Here's how the part is built. I have some questions about the finished solid (model axes, mm). Coordinates: 2 decimals unless noted, no trailing zeros. Write each loop counter-clockwise with the first axis right and the second up, starting at its lowest first coordinate (ties: lowest second). Pieces come first, ordered by that corner, then holes. Notation, with made-up numbers: M -17.75,-4.75 L -1.75,-4.75 A33 ccw -1.75,28.25 Z; hole C 63,69.5 d7. An arc over 180 degrees is marked long. Use a Markdown table: item, result.
```python
from build123d import *

# Parameters (mm, degrees)
F0_R     = 30
F0_R_2   = 2.5
F1_DEPTH = 6


with BuildPart() as f1:
    # F0 (on Top) → F1 (new body)
    with BuildSketch(Plane.XY):
        Circle(F0_R)
        with Locations((-11.5, -8.75)):
            Circle(F0_R_2, mode=Mode.SUBTRACT)
        with Locations((0, -8.75)):
            Circle(F0_R_2, mode=Mode.SUBTRACT)
        with Locations((11.5, -8.75)):
            Circle(F0_R_2, mode=Mode.SUBTRACT)
        with Locations((-11.5, 8.75)):
            Circle(F0_R_2, mode=Mode.SUBTRACT)
        with Locations((0, 8.75)):
            Circle(F0_R_2, mode=Mode.SUBTRACT)
        with Locations((11.5, 8.75)):
            Circle(F0_R_2, mode=Mode.SUBTRACT)
    extrude(amount=F1_DEPTH)


solid = f1.part
```
1. Suppose I cut it at D-D on x = 13. Write out the boundary of the cut face in (y, z), and give its area (3 significant figures).
Answers follow:
| item | result |
|---|---|
| outline | M -27.04,0 L -10.75,0 L -10.75,6 L -27.04,6 Z; M -6.75,0 L 6.75,0 L 6.75,6 L -6.75,6 Z; M 10.75,0 L 27.04,0 L 27.04,6 L 10.75,6 Z |
| area | 276 mm2 |
2. I need wall thicknesses on probe 1 along Y at (x, z) = (0, 3.6); probe 2 along X at (y, z) = (8, 0.8); probe 3 along Y at (x, z) = (-9.5, 3.6). Which ranges of each line are inside material? Lowest first, please.
Answers follow:
| item | result |
|---|---|
| probe 1 | y = -30 to -11.25, -6.25 to 6.25, 11.25 to 30 |
| probe 2 | x = -28.91 to -13.88, -9.12 to -2.38, 2.38 to 9.12, 13.88 to 28.91 |
| probe 3 | y = -28.46 to -10.25, -7.25 to 7.25, 10.25 to 28.46 |
3. Will these pins go through, and if not, where does the flat tip stop? pin 1 Ø2 at (y, z) = (-18, 4) entering from -X; pin 2 Ø4.5 at (x, y) = (11.5, -8.75) entering from -Z; pin 3 Ø3 at (x, z) = (-19.5, 5) entering from -Y.
Answers follow:
| item | result |
|---|---|
| pin 1 | stops at x = -24.72 |
| pin 2 | passes through |
| pin 3 | stops at y = -24 |
4. We'd pull the mould along Y, two halves only. Please class faces 1 (the face through (-29.97, 1.32, 2.96)), 2 (the face through (0, 0, 6)), 3 (the face through (11, 6.3, 3)): +Y half, -Y half, draft (parallel to the pull), parting line (faces both ways), or undercut.
Answers follow:
| item | result |
|---|---|
| face 1 | parting line |
| face 2 | draft |
| face 3 | undercut |
5. Suppose I cut it at C-C on y = -8.75. Write out the boundary of the cut face in (x, z).
Answers follow:
| item | result |
|---|---|
| outline | M -28.7,0 L -14,0 L -14,6 L -28.7,6 Z; M -9,0 L -2.5,0 L -2.5,6 L -9,6 Z; M 2.5,0 L 9,0 L 9,6 L 2.5,6 Z; M 14,0 L 28.7,0 L 28.7,6 L 14,6 Z |
6. Suppose I cut it at B-B on z = 2.2. Write out the boundary of the cut face in (x, y), and give its area (3 significant figures).
Answers follow:
| item | result |
|---|---|
| outline | C 0,0 d60; hole C -11.5,-8.75 d5; hole C -11.5,8.75 d5; hole C 0,-8.75 d5; hole C 0,8.75 d5; hole C 11.5,-8.75 d5; hole C 11.5,8.75 d5 |
| area | 2,710 mm2 |
7. Suppose I cut it at A-A on x = 0. Write out the boundary of the cut face in (y, z), and give its area (3 significant figures).
Answers follow:
| item | result |
|---|---|
| outline | M -30,0 L -11.25,0 L -11.25,6 L -30,6 Z; M -6.25,0 L 6.25,0 L 6.25,6 L -6.25,6 Z; M 11.25,0 L 30,0 L 30,6 L 11.25,6 Z |
| area | 300 mm2 |
